from build123d import *

# Parameters (mm, degrees)
REVOLUTION_ANGLE = 270


with BuildPart() as part:
    # Sketch → Revolution (revolve)
    with BuildSketch(Plane.XZ):
        Polygon((-45, 30), (45, 30), (45, 45), (7.5, 45), (7.5, 95), (35, 95), (45, 140), (35, 140), (28.333333, 110), (20.597845, 110), (5, 140), (-5, 140), (-20.597845, 110), (-28.333333, 110), (-35, 140), (-45, 140), (-35, 95), (-7.5, 95), (-7.5, 45), (-45, 45), align=None)
    revolve(axis=Axis((0, 0, 0), (1, 0, 0)), revolution_arc=REVOLUTION_ANGLE)


solid = part.part
Input: part model. Units: mm. Frame: model coordinates. A direction names the side the tool comes from. Coordinates: 2 decimals unless noted, no trailing zeros. Loops run counter-clockwise (first coordinate to the right, second up) from the corner with the lowest first, then second, coordinate; pieces in that order, holes last. Notation, with made-up numbers: (40.25, 51) -> (86.25, 51) arc R32 cw to (86.25, 79) -> close; hole circle Ø1 at (25, 64). An arc over 180 degrees is marked (long way). Write item = value, one per line. Start each with the question number.
Item 1: Reachability of faces 1 (the face through (7.5, -22, -41)), 2 (the face through (28.657, -81.368, -76.17)), 3 (the face through (-26.512, -32.852, -30.753)) from +Z, -Z, +X, -X, +Y, -Y: full face, straight path, thin tool, end or side. Return the list, or none.
Item 2: First-contact query: P1, Ø6, axis at x = 0.5, z = -84.5, coming from the -Y side; P2, Ø3, axis at y = -72.5, z = -90, coming from the +X side; P3, Ø3, axis at x = 21.5, y = -40, coming from the -Z side. Flat tips, straight axial feed; report the tip coordinate or a pass-through.
Item 3: Cut plane B-B, the plane z = -119. Count the separate pieces of the cut face and the enclosed holes in it, plus the area to 3 significant figures.
Item 4: Material intervals for line 1 (Z direction, x = 27.5, y = -34); line 2 (X direction, y = -108, z = 55); line 3 (X direction, y = -57.5, z = -19), sorted ascending.
Item 5: Cut plane C-C, the plane x = 0. Return loops of the section in (y, z), plus the area to 3 significant figures.
Item 6: Mould query, pull axis Y, two halves, no side actions, for faces 4 (the face through (-1, 0, 86)), 5 (the face through (21.443, -69.354, -64.923)), 6 (the face through (-24.52, -80.305, -75.174)), 7 (the face through (45, -20, -23)). Classes: pulls with the +Y half, pulls with the -Y half, needs draft (parallel to the pull), parting line crosses it, or undercut.
Item 7: Cut plane A-A, the plane x = 25. Return loops of the section in (y, z), plus the area to 3 significant figures.
Ans:
q1.face_1 = +X
q1.face_2 = none
q1.face_3 = -X
q2.P1 = -113.83
q2.P2 = 39.9
q2.P3 = -103.76
q3.separate_pieces = 3
q3.enclosed_holes = 0
q3.area = 6,540 mm²
q4.line_1 = -104.61 to -88.71, -29.48 to 29.48, 88.71 to 104.61
q4.line_2 = -40.82 to -30.82, -14.78 to 14.78, 30.82 to 40.82
q4.line_3 = -7.5 to 7.5
q5.outline = (0, 30) -> (0, 140) arc R140 ccw (long way) to (140, 0) -> (30, 0) arc R30 cw (long way) to start
q5.area = 44,100 mm²
q6.face_4 = pulls with the +Y half
q6.face_5 = undercut
q6.face_6 = parting line crosses it
q6.face_7 = needs draft
q7.outline = (0, 30) -> (0, 45) arc R45 ccw (long way) to (45, 0) -> (30, 0) arc R30 cw (long way) to start; (0, 95) -> (0, 110) arc R110 ccw (long way) to (110, 0) -> (95, 0) arc R95 cw (long way) to start
q7.area = 9,900 mm²
